Geometry: final body of the model. Coordinates: model frame, mm. A direction names the side the tool comes from. Round coordinates to 2 decimals unless told otherwise and drop trailing zeros. Write each loop counter-clockwise with the first axis right and the second up, starting at its lowest first coordinate (ties: lowest second). Pieces come first, ordered by that corner, then holes. Notation, with made-up numbers: M -7,42.5 L 34,42.5 A11 ccw 34,55.5 Z; hole C 89.25,72 d7. An arc over 180 degrees is marked long. Answer as CSV lines item,"result". Start each with the question number.
Q1. Reachability of faces 1 (the flat face through (-49, 19, 1)), 2 (the flat face through (-114, 37, -27.008)), 3 (the flat face through (-79, 5, 0)) from +Z, -Z, +X, -X, +Y, -Y: full face, straight path, thin tool, end or side. Return the list, or none.
Q2. First-contact query: pin 1 (10 mm diameter, centred on x = -85.5, y = 15.5, fed in from +Z); pin 2 (24.5 mm diameter, centred on x = -62, z = 33.5, fed in from +Y); pin 3 (18.5 mm diameter, centred on x = -50.5, z = -41.5, fed in from +Y). Flat tips, straight axial feed; report the tip coordinate or a pass-through.
Q3. Section query B-B on x = -82.5. Output: boundary loops of the cut face in (y, z), and give its area (3 significant figures).
Q4. Section query A-A on z = 41. Output: boundary loops of the cut face in (x, y), and give its area (3 significant figures).
Q5. Section query C-C on y = 41.5. Output: boundary loops of the cut face in (x, z), and give its area (3 significant figures).
Q6. Ray query, probe 1 along Y at (x, z) = (-31, 30); probe 2 along Z at (x, y) = (-144, 56); probe 3 along X at (y, z) = (42, -6.5). Return the intervals inside material, ascending.
Q7. Section query D-D on z = -11.5. Output: boundary loops of the cut face in (x, y), and give its area (3 significant figures).
Q8. Mould query, pull axis Y, two halves, no side actions, for faces 4 (the flat face through (-130, 19, 38)), 5 (the flat face through (-79, -5, 38)), 6 (the flat face through (-130, 49, 48.992)). Classes: pulls with the +Y half, pulls with the -Y half, needs draft (parallel to the pull), parting line crosses it, or undercut.
```python
from build123d import *

# Parameters (mm, degrees)
BOSS_EXTRUDE1_DEPTH = 160
SKETCH2_R           = 15
BOSS_EXTRUDE2_DEPTH = 76


with BuildPart() as part:
    # Sketch1 → Boss-Extrude1 (new body)
    with BuildSketch(Plane(origin=(0, 0, 0), x_dir=(0, 0, -1), z_dir=(1, 0, 0))):
        Polygon((-26, -5), (-50, -5), (-50, 7), (-27.572519084, 7), (-27.572519084, 19), (27.007633588, 19), (27.007633588, 9.076335878), (50, 9.076335878), (50, -5), (26, -5), (26, 5), (-26, 5), align=None)
    extrude(amount=-BOSS_EXTRUDE1_DEPTH)

    # Sketch2 → Boss-Extrude2 (add)
    with BuildSketch(Plane(origin=(0, 0, -27.007633588), x_dir=(-1, 0, 0), z_dir=(0, 0, -1))):
        with BuildLine():
            Line((100, 19), (160, 19))
            Line((160, 19), (160, 49))
            ThreePointArc((160, 49), (130, 79), (100, 49))
            Line((100, 49), (100, 19))
        make_face()
        with Locations((130, 49)):
            Circle(SKETCH2_R, mode=Mode.SUBTRACT)
        with Locations((130, 49)):
            Circle(SKETCH2_R)
    extrude(amount=-BOSS_EXTRUDE2_DEPTH)


solid = part.part
```
Entries:
1,face 1,"+Z, -Z, +X, +Y"
1,face 2,"-Z, +X, -X, +Y"
1,face 3,"+X, -X, -Y"
2,pin 1,"stops at z = 27.57"
2,pin 2,"stops at y = 19"
2,pin 3,"stops at y = 9.08"
3,outline,"M -5,-50 L 9.08,-50 L 9.08,-27.01 L 19,-27.01 L 19,27.57 L 7,27.57 L 7,50 L -5,50 L -5,26 L 5,26 L 5,-26 L -5,-26 Z"
3,area,"1,380 mm^2"
4,outline,"M -160,-5 L 0,-5 L 0,7 L -160,7 Z; M -160,19 L -100,19 L -100,49 A30 ccw -160,49 Z"
4,area,"5,130 mm^2"
5,outline,"M -160,-27.01 L -100,-27.01 L -100,48.99 L -160,48.99 Z"
5,area,"4,560 mm^2"
6,probe 1,"y = -5 to 7"
6,probe 2,"z = -27.01 to 48.99"
6,probe 3,"x = -160 to -100"
7,outline,"M -160,5 L 0,5 L 0,19 L -100,19 L -100,49 A30 ccw -160,49 Z"
7,area,"5,450 mm^2"
8,face 4,"undercut"
8,face 5,"pulls with the -Y half"
8,face 6,"needs draft"
